```python
from build123d import *

# Parameters (mm, degrees)
SKETCH1_W                        = 26.416
SKETCH1_H                        = 18.034
BOSS_EXTRUDE2_DEPTH              = 1.524
SKETCH1_4_W                      = 1.524
SKETCH1_4_H                      = 18.034
BOSS_EXTRUDE3_DEPTH              = 27.94
FILLET1_R                        = 1.27
FILLET2_R                        = 6.35
F_10_0_1935_DIAMETER_HOLE1_D     = 4.9149
F_10_0_1935_DIAMETER_HOLE1_DEPTH = 5.08
F_10_0_1935_DIAMETER_HOLE1_TIP   = 1.476584928
F_10_0_1935_DIAMETER_HOLE2_D     = 4.9149
F_10_0_1935_DIAMETER_HOLE2_DEPTH = 5.08
F_10_0_1935_DIAMETER_HOLE2_TIP   = 1.476584928


with BuildPart() as part:
    # Sketch1 → Boss-Extrude2 (new body)
    with BuildSketch(Plane(origin=(0, 0, 0), x_dir=(1, 0, 0), z_dir=(0, 1, 0))):
        with Locations((1.735252818, 0.105208004)):
            Rectangle(SKETCH1_W, SKETCH1_H)
    extrude(amount=BOSS_EXTRUDE2_DEPTH)

    # Sketch1<4> → Boss-Extrude3 (add)
    with BuildSketch(Plane(origin=(0, 0, 0), x_dir=(1, 0, 0), z_dir=(0, 1, 0))):
        with Locations((-12.234747182, 0.105208004)):
            Rectangle(SKETCH1_4_W, SKETCH1_4_H)
    extrude(amount=BOSS_EXTRUDE3_DEPTH)

    # Fillet1
    fillet1_edges = [part.edges().sort_by_distance(p)[0] for p in [
        (-12.996747182, 0, -0.105208004),
        (-11.472747182, 1.524, -0.105208004),
    ]]
    fillet(fillet1_edges, radius=FILLET1_R)

    # Fillet2
    fillet2_edges = [part.edges().sort_by_distance(p)[0] for p in [
        (-12.234747182, 27.94, -9.122208004),
        (-12.234747182, 27.94, 8.911791996),
        (14.943252818, 0.762, 8.911791996),
        (14.943252818, 0.762, -9.122208004),
    ]]
    fillet(fillet2_edges, radius=FILLET2_R)

    # #10 (0.1935) Diameter Hole1
    with Locations(Plane(origin=(0, 1.524, 0), x_dir=(1, 0, 0), z_dir=(0, 1, 0))):
        with Locations((-3.852747182, 0.105208004), (8.085252818, 0.105208004)):
            Hole(F_10_0_1935_DIAMETER_HOLE1_D / 2, depth=F_10_0_1935_DIAMETER_HOLE1_DEPTH)
            with Locations((0, 0, -(F_10_0_1935_DIAMETER_HOLE1_DEPTH + F_10_0_1935_DIAMETER_HOLE1_TIP / 2))):  # 118° drill point
                Cone(0, F_10_0_1935_DIAMETER_HOLE1_D / 2, F_10_0_1935_DIAMETER_HOLE1_TIP, mode=Mode.SUBTRACT)

    # #10 (0.1935) Diameter Hole2
    with Locations(Plane(origin=(-11.472747182, 0, 0), x_dir=(0, 0, -1), z_dir=(1, 0, 0))):
        with Locations((0.105208004, 9.144), (0.105208004, 21.082)):
            Hole(F_10_0_1935_DIAMETER_HOLE2_D / 2, depth=F_10_0_1935_DIAMETER_HOLE2_DEPTH)
            with Locations((0, 0, -(F_10_0_1935_DIAMETER_HOLE2_DEPTH + F_10_0_1935_DIAMETER_HOLE2_TIP / 2))):  # 118° drill point
                Cone(0, F_10_0_1935_DIAMETER_HOLE2_D / 2, F_10_0_1935_DIAMETER_HOLE2_TIP, mode=Mode.SUBTRACT)


solid = part.part
```
The model under review builds one solid part; all positions refer to its coordinate system, in mm. A direction names the side the tool comes from. Round coordinates to 2 decimals unless told otherwise and drop trailing zeros. Write each loop counter-clockwise with the first axis right and the second up, starting at its lowest first coordinate (ties: lowest second). Pieces come first, ordered by that corner, then holes.
(1) We need section B-B on x = -4.5. Give the boundary of the cut face in (y, z).
(2) Insertion check: pin 1 (4 mm diameter, centred on x = 11.5, z = 2.5, fed in from +Y); pin 2 (8 mm diameter, centred on y = 21.08, z = -0.11, fed in from +X). Each pin has a flat end and moves straight along its axis. Give the tip position at first contact, or say it passes through.
(3) Mouldability with a two-part tool opening along X and no side actions: class faces 1 (the flat face through (-12, 6, -9.122)), 2 (the cylindrical face through (13.034, 0.773, -7.311)), 3 (the cylindrical face through (5.74, 0.75, -0.84)) as +X half, -X half, draft (parallel to the pull), parting line (faces both ways), or undercut.
(4) Wall thickness on L1, parallel to X at y = 22.5, z = 6.75; L2, parallel to Y at x = -2.75, z = 4.75: over which ranges is each line inside the solid? List them lowest first.
(5) We need section D-D on y = 13. Give the boundary of the cut face in (x, z), and give its area (3 significant figures).
(6) Machinability: for faces 4 (the cylindrical face through (-12.245, 11.216, 1.216)), 5 (the flat face through (2, 1.524, 0)), which of the approach directions +Z, -Z, +X, -X, +Y, -Y give a long, thin tool a straight path to every point of the face, cutting with its end or side? Answer none if there is none.
(7) We need section C-C on z = -4.25. Give the boundary of the cut face in (x, y).
(8) We need section A-A on z = -1.75. Give the boundary of the cut face in (x, y).
Findings below:
1. outline: (0, -9.12) - (1.52, -9.12) - (1.52, -2.48) - (0, -2.48) - close; (0, 2.27) - (1.52, 2.27) - (1.52, 8.91) - (0, 8.91) - close
2. pin 1: stops at y = 1.52
2. pin 2: stops at x = -11.47
3. face 1: draft
3. face 2: +X half
3. face 3: undercut
4. L1: x = -13 to -11.47
4. L2: y = 0 to 1.52
5. outline: (-13, -9.12) - (-11.47, -9.12) - (-11.47, 8.91) - (-13, 8.91) - close
5. area: 27.5 mm2
6. face 4: +X, -X
6. face 5: +Z, -Z, +X, +Y
7. outline: (-13, 1.27) arc R1.27 ccw to (-11.73, 0) - (14.77, 0) - (14.77, 1.52) - (-10.2, 1.52) arc R1.27 cw to (-11.47, 2.79) - (-11.47, 27.77) - (-13, 27.77) - close
8. outline: (-13, 1.27) arc R1.27 ccw to (-11.73, 0) - (-5.68, 0) - (-5.68, 1.52) - (-10.2, 1.52) arc R1.27 cw to (-11.47, 2.79) - (-11.47, 7.32) - (-13, 7.32) - close; (-13, 10.97) - (-11.47, 10.97) - (-11.47, 19.26) - (-13, 19.26) - close; (-13, 22.91) - (-11.47, 22.91) - (-11.47, 27.94) - (-13, 27.94) - close; (-2.03, 0) - (6.26, 0) - (6.26, 1.52) - (-2.03, 1.52) - close; (9.91, 0) - (14.94, 0) - (14.94, 1.52) - (9.91, 1.52) - close
